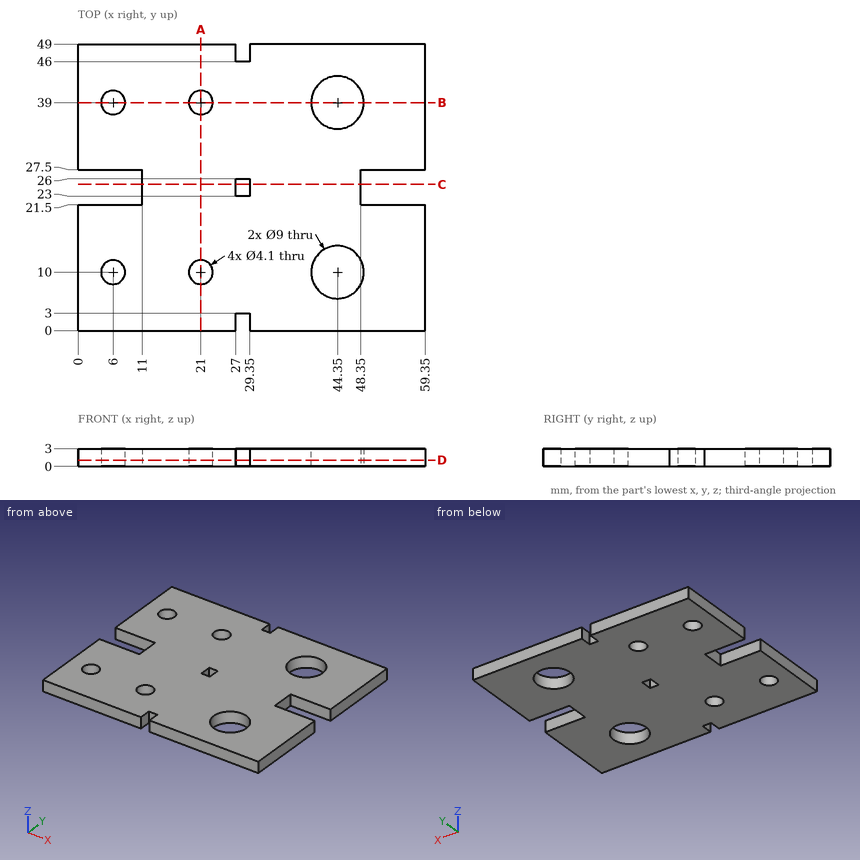
Could you check a few things on this drawing? It's one solid part, dimensions in mm from its lowest x, y, z. Coordinates: 2 decimals unless noted, no trailing zeros. Order: outer loops, then holes, each group sorted by start corner. A loop starts at its lowest first (then second) coordinate and runs counter-clockwise, first axis right, second up.
1) Will these pins go through, and if not, where does the flat tip stop? pin 1 (5.5 mm diameter, centred on x = 44.35, y = 39, fed in from +Z); pin 2 (0.7 mm diameter, centred on x = 27.5, z = 2, fed in from +Y); pin 3 (1.5 mm diameter, centred on y = 24.5, z = 2, fed in from -X).
2) Imagine slicing it at A-A on x = 21. List the corners of the cut face in (y, z) for me, and give its area (3 significant figures).
3) Imagine slicing it at B-B on y = 39. List the corners of the cut face in (x, z) for me, and give its area (3 significant figures).
4) Imagine slicing it at C-C on y = 25. List the corners of the cut face in (x, z) for me, and give its area (3 significant figures).
5) I need wall thicknesses on line 1 (Y direction, x = 44.5, z = 0.5); line 2 (Y direction, x = 21, z = 0.9); line 3 (Y direction, x = 6, z = 1.5). Which ranges of each line are inside material? Lowest first, please.
6) Imagine slicing it at D-D on z = 1.05. State how many separate pieces and enclosed holes the cut face has, and give its area (3 significant figures).
Response values:
1. pin 1: passes through
1. pin 2: stops at y = 46
1. pin 3: stops at x = 11
2. outline: (0, 0) - (7.95, 0) - (7.95, 3) - (0, 3) - close; (12.05, 0) - (36.95, 0) - (36.95, 3) - (12.05, 3) - close; (41.05, 0) - (49, 0) - (49, 3) - (41.05, 3) - close
2. area: 122 mm2
3. outline: (0, 0) - (3.95, 0) - (3.95, 3) - (0, 3) - close; (8.05, 0) - (18.95, 0) - (18.95, 3) - (8.05, 3) - close; (23.05, 0) - (39.85, 0) - (39.85, 3) - (23.05, 3) - close; (48.85, 0) - (59.35, 0) - (59.35, 3) - (48.85, 3) - close
3. area: 126 mm2
4. outline: (11, 0) - (27, 0) - (27, 3) - (11, 3) - close; (29.35, 0) - (48.35, 0) - (48.35, 3) - (29.35, 3) - close
4. area: 105 mm2
5. line 1: y = 0 to 5.5, 14.5 to 34.5, 43.5 to 49
5. line 2: y = 0 to 7.95, 12.05 to 36.95, 41.05 to 49
5. line 3: y = 0 to 7.95, 12.05 to 21.5, 27.5 to 36.95, 41.05 to 49
6. separate pieces: 1
6. enclosed holes: 7
6. area: 2,570 mm2
